Verification items for the finished model (mm, model axes). Face numbers are marked on the shaded views. A direction names the side the tool comes from. Give positions to 0.01 mm unless a question says otherwise; leave off trailing zeros. Order: outer loops, then holes, each group sorted by start corner. A loop starts at its lowest first (then second) coordinate and runs counter-clockwise, first axis right, second up.
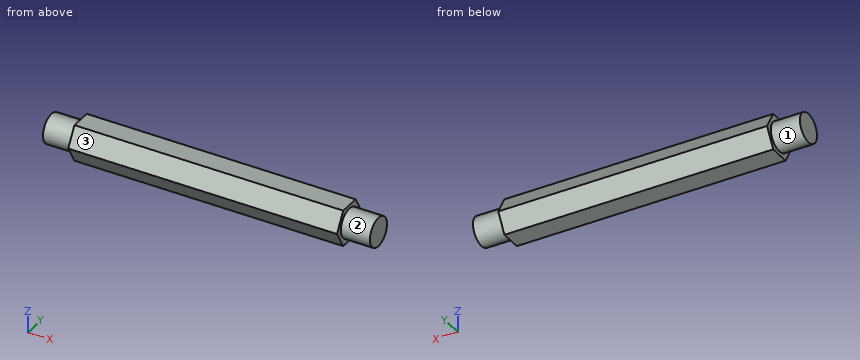
from build123d import *

# Parameters (mm, degrees)
BOSS_EXTRUDE1_DEPTH = 37


with BuildPart() as part:
    # Sketch1 → Revolve1 (revolve)
    with BuildSketch(Plane.XY):
        Polygon((0, 2), (-4, 2), (-4, 0), (41, 0), (41, 2), (37, 2), (37, 2.5), (0, 2.5), align=None)
    revolve(axis=Axis((-6.185185185, 0, 0), (1, 0, 0)))

    # Sketch2 → Boss-Extrude1 (add)
    with BuildSketch(Plane(origin=(0, 0, 0), x_dir=(0, 0, -1), z_dir=(1, 0, 0))):
        Polygon((0, 2.886751346), (-2.5, 1.443375673), (-2.5, -1.443375673), (0, -2.886751346), (2.5, -1.443375673), (2.5, 1.443375673), align=None)
    extrude(amount=BOSS_EXTRUDE1_DEPTH)


solid = part.part
(1) Go/stop test with flat-tipped pins: pin 1 (2 mm diameter, centred on x = 15, z = 0.5, fed in from -Y); pin 2 (2 mm diameter, centred on x = 22, z = -0.5, fed in from +Y). Record where each tip stops, or that it passes through.
Solved:
pin 1: stops at y = -2.89
pin 2: stops at y = 2.89
(2) Section check C-C, the plane y = 0. Enter the section's corners in (x, z), then the cut area to 3 significant figures.
Solved:
outline: (-4, -2) - (0, -2) - (0, -2.5) - (37, -2.5) - (37, -2) - (41, -2) - (41, 2) - (37, 2) - (37, 2.5) - (0, 2.5) - (0, 2) - (-4, 2) - close
area: 217 mm2
(3) Section check A-A, the plane x = 16. Enter the section's corners in (y, z).
Solved:
outline: (-2.89, 0) - (-1.44, -2.5) - (1.44, -2.5) - (2.89, 0) - (1.44, 2.5) - (-1.44, 2.5) - close
(4) Section check B-B, the plane z = -0.55. Enter the section's corners in (x, y).
Solved:
outline: (-4, -1.92) - (0, -1.92) - (0, -2.57) - (37, -2.57) - (37, -1.92) - (41, -1.92) - (41, 1.92) - (37, 1.92) - (37, 2.57) - (0, 2.57) - (0, 1.92) - (-4, 1.92) - close
(5) Scan lines: line 1 (X direction, y = 1.2, z = -1.95); line 2 (Y direction, x = 36, z = -0.5); line 3 (Z direction, x = 7.5, y = 2.5). Record each from-to range of solid material in increasing order.
Solved:
line 1: x = 0 to 37
line 2: y = -2.6 to 2.6
line 3: z = -0.67 to 0.67
(6) Set-up check for the marked faces 1, 2 and 3: record each of +Z, -Z, +X, -X, +Y, -Y from which the full face is reachable in a straight line by a thin tool's end or side.
Solved:
face 1: -X
face 2: +X
face 3: +Z, +X, -X, -Y
(7) Section check D-D, the plane x = 37.5. Enter the section's corners in (y, z), then the cut area to 3 significant figures.
Solved:
outline: circle Ø4 at (0, 0)
area: 12.6 mm2
